Build history of the part. All positions in model axes, mm. A direction names the side the tool comes from. Round coordinates to 2 decimals unless told otherwise and drop trailing zeros. Loops run counter-clockwise (first coordinate to the right, second up) from the corner with the lowest first, then second, coordinate; pieces in that order, holes last. Notation, with made-up numbers: (55.25, 88) -> (108.25, 88) arc R13 ccw to (108.25, 100) -> close; hole circle Ø11 at (-1, 12.5). An arc over 180 degrees is marked (long way). Put each result on its own line as item: value. Start each with the question number.
Item 1: Cut at A-A, the plane x = 20. List the corners of the cut face in (y, z).
Item 2: Tool access for faces 4 (the flat face through (32, 0, 1)), 5 (the flat face through (0, 5, -1)), 6 (the flat face through (0, -7, 23.25)), 7 (the flat face through (-22.305, 8.606, 0.595)): list every direction of +Z, -Z, +X, -X, +Y, -Y with a clear straight run to the whole face (end or side of a thin tool).
Item 3: Cut at D-D, the plane x = -8.5. List the corners of the cut face in (y, z).
Item 4: Flat gauge pins, fed straight in: pin 1 Ø4 at (x, z) = (-6, -5) entering from +Y; pin 2 Ø5 at (y, z) = (3.5, 17.5) entering from -X; pin 3 Ø3 at (x, z) = (-18, -10) entering from +Y. Where does each tip first touch, or does it go through?
Item 5: Pull direction X, two halves, no side cores. Call faces 1 (the flat face through (-1, -8, 29)), 2 (the cylindrical face through (-30.33, -3.04, 21.14)), 3 (the flat face through (-25, 5, 1)): +X half, -X half, draft (parallel to the pull), parting line (faces both ways), or undercut.
Item 6: Drill centre lines: probe 1 along Z at (x, y) = (-30, -2.55); probe 2 along X at (y, z) = (8.25, 23.5); probe 3 along Y at (x, z) = (6, -19). Where is each one in solid material? Low to high. Write a range as [from, to].
Item 7: Cut at C-C, the plane y = 1.5. List the corners of the cut face in (x, z), plus the area to 3 significant figures.
Item 8: Cut at B-B, the plane z = 7.5. List the corners of the cut face in (x, y).
```python
from build123d import *

# Parameters (mm, degrees)
SKETCH7_W           = 50
SKETCH7_H           = 85
BOSS_EXTRUDE5_DEPTH = 10
SKETCH8_W           = 28
SKETCH8_H           = 85
CUT_EXTRUDE1_DEPTH  = 5
SKETCH11_W          = 11
SKETCH11_H          = 85
BOSS_EXTRUDE6_DEPTH = 3.5
CUT_EXTRUDE5_DEPTH  = 86
CUT_EXTRUDE6_DEPTH  = 86
SKETCH14_W          = 50
SKETCH14_H          = 85
SKETCH14_W_2        = 15
BOSS_EXTRUDE7_DEPTH = 8
CUT_EXTRUDE11_DEPTH = 2
SKETCH19_R          = 2.510624494
CUT_EXTRUDE12_DEPTH = 20.5


with BuildPart() as part:
    # Sketch7 → Boss-Extrude5 (new body)
    with BuildSketch(Plane(origin=(0, 0, 0), x_dir=(1, 0, 0), z_dir=(0, 1, 0))):
        Rectangle(SKETCH7_W, SKETCH7_H)
    extrude(amount=BOSS_EXTRUDE5_DEPTH)

    # Sketch8 → Cut-Extrude1 (cut)
    with BuildSketch(Plane(origin=(0, 10, 0), x_dir=(1, 0, 0), z_dir=(0, 1, 0))):
        Rectangle(SKETCH8_W, SKETCH8_H)
    extrude(amount=-CUT_EXTRUDE1_DEPTH, mode=Mode.SUBTRACT)

    # Sketch11 → Boss-Extrude6 (add)
    with BuildSketch(Plane(origin=(0, 10, 0), x_dir=(1, 0, 0), z_dir=(0, 1, 0))):
        with Locations((19.5, 0)):
            Rectangle(SKETCH11_W, SKETCH11_H)
    extrude(amount=BOSS_EXTRUDE6_DEPTH)

    # Sketch12 → Cut-Extrude5 (cut, through all)
    with BuildSketch(Plane.XY.offset(42.5)):
        with BuildLine():
            Line((-21.5, 10), (-17.5, 10))
            Line((-17.5, 10), (-15.91228676, 7.25))
            ThreePointArc((-15.91228676, 7.25), (-15.91228676, 6.75), (-16.345299462, 6.5))
            Line((-16.345299462, 6.5), (-22.654700538, 6.5))
            ThreePointArc((-22.654700538, 6.5), (-23.08771324, 6.75), (-23.08771324, 7.25))
            Line((-23.08771324, 7.25), (-21.5, 10))
        make_face()
    extrude(amount=-CUT_EXTRUDE5_DEPTH, mode=Mode.SUBTRACT)

    # Sketch13 → Cut-Extrude6 (cut, through all)
    with BuildSketch(Plane.XY.offset(42.5)):
        with BuildLine():
            Line((21.5, 10), (25, 10))
            Line((25, 10), (25, 13.5))
            Line((25, 13.5), (22.654700538, 13.5))
            ThreePointArc((22.654700538, 13.5), (23.08771324, 13.25), (23.08771324, 12.75))
            Line((23.08771324, 12.75), (21.5, 10))
        make_face()
        with BuildLine():
            Line((14, 10), (17.5, 10))
            Line((17.5, 10), (15.91228676, 12.75))
            ThreePointArc((15.91228676, 12.75), (15.91228676, 13.25), (16.345299462, 13.5))
            Line((16.345299462, 13.5), (14, 13.5))
            Line((14, 13.5), (14, 10))
        make_face()
    extrude(amount=-CUT_EXTRUDE6_DEPTH, mode=Mode.SUBTRACT)

    # Sketch14 → Boss-Extrude7 (add)
    with BuildSketch(Plane.XZ):
        Rectangle(SKETCH14_W, SKETCH14_H)
        with Locations((32.5, 0)):
            Rectangle(SKETCH14_W_2, SKETCH14_H)
        with Locations((-32.5, 0)):
            Rectangle(SKETCH14_W_2, SKETCH14_H)
    extrude(amount=BOSS_EXTRUDE7_DEPTH)

    # Sketch18 → Cut-Extrude11 (cut)
    with BuildSketch(Plane.XZ.offset(8)):
        with BuildLine():
            Line((30.5, -23.25), (-30.5, -23.25))
            ThreePointArc((-30.5, -23.25), (-33.399137803, -22.049137803), (-34.6, -19.15))
            Line((-34.6, -19.15), (-34.6, 19.15))
            ThreePointArc((-34.6, 19.15), (-33.399137803, 22.049137803), (-30.5, 23.25))
            Line((-30.5, 23.25), (30.5, 23.25))
            ThreePointArc((30.5, 23.25), (33.399137803, 22.049137803), (34.6, 19.15))
            Line((34.6, 19.15), (34.6, -19.15))
            ThreePointArc((34.6, -19.15), (33.399137803, -22.049137803), (30.5, -23.25))
        make_face()
    extrude(amount=-CUT_EXTRUDE11_DEPTH, mode=Mode.SUBTRACT)

    # Sketch19 → Cut-Extrude12 (cut, through all)
    with BuildSketch(Plane.XZ.offset(6)):
        with Locations((-30, 18.65)):
            Circle(SKETCH19_R)
        with Locations((-30, -18.65)):
            Circle(SKETCH19_R)
        with Locations((30, -18.65)):
            Circle(SKETCH19_R)
        with Locations((30, 18.65)):
            Circle(SKETCH19_R)
    extrude(amount=-CUT_EXTRUDE12_DEPTH, mode=Mode.SUBTRACT)


solid = part.part
```
Reply:
1. outline: (-8, -42.5) -> (13.5, -42.5) -> (13.5, 42.5) -> (-8, 42.5) -> (-8, 23.25) -> (-6, 23.25) -> (-6, -23.25) -> (-8, -23.25) -> close
2. face 4: +Z, -Z, +X, +Y
2. face 5: +Z, -Z, +Y
2. face 6: -Y
2. face 7: +Z, -Z
3. outline: (-8, -42.5) -> (5, -42.5) -> (5, 42.5) -> (-8, 42.5) -> (-8, 23.25) -> (-6, 23.25) -> (-6, -23.25) -> (-8, -23.25) -> close
4. pin 1: stops at y = 5
4. pin 2: stops at x = -25
4. pin 3: stops at y = 10
5. face 1: draft
5. face 2: undercut
5. face 3: -X half
6. probe 1: z = [-42.5, -21.16], [-16.14, 16.14], [21.16, 42.5]
6. probe 2: x = [-25, -22.51], [-16.49, -14], [14, 25]
6. probe 3: y = [-6, 5]
7. outline: (-25, -42.5) -> (25, -42.5) -> (25, 42.5) -> (-25, 42.5) -> close
7. area: 4,250 mm^2
8. outline: (-40, -8) -> (-34.6, -8) -> (-34.6, -6) -> (34.6, -6) -> (34.6, -8) -> (40, -8) -> (40, 0) -> (25, 0) -> (25, 10) -> (21.5, 10) -> (23.09, 12.75) arc R0.5 ccw to (22.65, 13.5) -> (16.35, 13.5) arc R0.5 ccw to (15.91, 12.75) -> (17.5, 10) -> (14, 10) -> (14, 5) -> (-14, 5) -> (-14, 10) -> (-17.5, 10) -> (-15.91, 7.25) arc R0.5 cw to (-16.35, 6.5) -> (-22.65, 6.5) arc R0.5 cw to (-23.09, 7.25) -> (-21.5, 10) -> (-25, 10) -> (-25, 0) -> (-40, 0) -> close
